Check sheet for the modelled part. Datum: model origin and axes. Units: mm. A direction names the side the tool comes from. Give positions to 0.01 mm unless a question says otherwise; leave off trailing zeros. Write each loop counter-clockwise with the first axis right and the second up, starting at its lowest first coordinate (ties: lowest second). Pieces come first, ordered by that corner, then holes. Notation, with made-up numbers: (37.5, 47.25) -> (73.5, 47.25) arc R26 ccw to (73.5, 76.25) -> close; hole circle Ø4 at (-40, -32.5). An arc over 180 degrees is marked (long way). Return JSON: item names as keys, results as strings.
from build123d import *

# Parameters (mm, degrees)
SKETCH_1_R          = 8
EXTRUDE_1_DEPTH     = 16
CUT_EXTRUDE_1_DEPTH = 8
CUT_EXTRUDE_2_DEPTH = 8


with BuildPart() as part:
    # 草图1 → 凸台-拉伸1 (new body)
    with BuildSketch(Plane.XY):
        Circle(SKETCH_1_R)
    extrude(amount=EXTRUDE_1_DEPTH)

    # 草图2 → 切除-拉伸1 (cut)
    with BuildSketch(Plane(origin=(0, 0, 0), x_dir=(-1, 0, 0), z_dir=(0, 0, -1))):
        with BuildLine():
            Line((3.020550217, 2.622265506), (3.020550217, -2.622265506))
            ThreePointArc((3.020550217, -2.622265506), (-4, 0), (3.020550217, 2.622265506))
        make_face()
    extrude(amount=-CUT_EXTRUDE_1_DEPTH, mode=Mode.SUBTRACT)

    # 草图3 → 切除-拉伸2 (cut)
    with BuildSketch(Plane.XY.offset(16)):
        with BuildLine():
            Line((-1.578947526, -1.938278801), (-1.578947526, 1.938278801))
            ThreePointArc((-1.578947526, 1.938278801), (2.5, 0), (-1.578947526, -1.938278801))
        make_face()
    extrude(amount=-CUT_EXTRUDE_2_DEPTH, mode=Mode.SUBTRACT)


solid = part.part
(1) Release check for a two-part mould opening along Y. For faces 4 (the flat face through (-2, 0, 16)), 5 (the flat face through (-3.021, 0, 4)), 6 (the cylindrical face through (-1.73, -7.81, 7.89)), 7 (the cylindrical face through (2.5, 0.1, 12.1)) record: pulls with the +Y half, pulls with the -Y half, needs draft (parallel to the pull), parting line crosses it, or undercut.
Reply:
{"face 4": "needs draft", "face 5": "undercut", "face 6": "parting line crosses it", "face 7": "undercut"}
(2) Set-up check for faces 1 (the flat face through (-1.579, 0, 12)), 2 (the flat face through (-4, 0, 0)), 3 (the flat face through (-2, 0, 8)): record each of +Z, -Z, +X, -X, +Y, -Y from which the full face is reachable in a straight line by a thin tool's end or side.
Reply:
{"face 1": "+Z, -Z", "face 2": "-Z, +X, -X, +Y, -Y", "face 3": "-Z"}
(3) Depth check by flat-ended pin: pin 1 Ø1 at (y, z) = (5.5, 7) entering from -X (3 decimals); pin 2 Ø1.5 at (x, z) = (2, 10) entering from -Y; pin 3 Ø2 at (y, z) = (-5.5, 13) entering from +X. Enter the tip coordinate at first touch or a pass-through.
Reply:
{"pin 1": "x = -6.245", "pin 2": "y = -7.9", "pin 3": "x = 6.61"}
(4) Cross-section at A-A on y = 0. Enter the section's corners in (x, z).
Reply:
{"outline": "(-8, 0) -> (-3.02, 0) -> (-3.02, 8) -> (-1.58, 8) -> (-1.58, 16) -> (-8, 16) -> close; (2.5, 8) -> (4, 8) -> (4, 0) -> (8, 0) -> (8, 16) -> (2.5, 16) -> close"}
(5) Cross-section at C-C on z = 2.75. Enter the section's corners in (x, y).
Reply:
{"outline": "circle Ø16 at (0, 0); hole (-3.02, -2.62) arc R4 ccw (long way) to (-3.02, 2.62) -> close"}
(6) Cross-section at B-B on x = 0. Enter the section's corners in (y, z).
Reply:
{"outline": "(-8, 0) -> (-4, 0) -> (-4, 8) -> (-2.5, 8) -> (-2.5, 16) -> (-8, 16) -> close; (2.5, 8) -> (4, 8) -> (4, 0) -> (8, 0) -> (8, 16) -> (2.5, 16) -> close"}
(7) Thickness scan on L1, parallel to Y at x = 0, z = 4.75; L2, parallel to Y at x = 0, z = 11.75; L3, parallel to Z at x = 2.75, y = -1.5. Record the ranges inside material, lowest first.
Reply:
{"L1": "-8 to -4, 4 to 8", "L2": "-8 to -2.5, 2.5 to 8", "L3": "8 to 16"}
(8) Cross-section at D-D on x = 3.75. Enter the section's corners in (y, z), then the cut area to 3 significant figures.
Reply:
{"outline": "(-7.07, 0) -> (-1.39, 0) -> (-1.39, 8) -> (1.39, 8) -> (1.39, 0) -> (7.07, 0) -> (7.07, 16) -> (-7.07, 16) -> close", "area": "204 mm^2"}
